```python
from build123d import *


with BuildPart() as f1:
    # F0 (on Front) → F1 (revolve)
    with BuildSketch(Plane.XZ):
        Polygon((0, 3.0734), (0, 0), (25.4, 0), (46.035527, 41.271053), (46.613301, 42.426601), (47.191074, 43.582149), (47.685844, 44.571688), (50.8, 50.8), (47.363834, 50.8), (23.500534, 3.0734), align=None)
        Polygon((47.191074, 43.582149), (46.613301, 42.426601), (47.191074, 42.426601), align=None)
        Polygon((47.685844, 44.571688), (47.191074, 43.582149), (47.685844, 43.582149), align=None)
        Polygon((46.613301, 42.426601), (46.035527, 41.271053), (46.613301, 41.271053), align=None)
    revolve(axis=Axis((0, 0, 25.4), (0, 0, 1)))


solid = f1.part
```
Model file for the job. Use its own axes, mm. A direction names the side the tool comes from. Coordinates: 2 decimals unless noted, no trailing zeros. Write each loop counter-clockwise with the first axis right and the second up, starting at its lowest first coordinate (ties: lowest second). Pieces come first, ordered by that corner, then holes. Notation, with made-up numbers: (-14.75, -26.75) - (3.25, -26.75) arc R16 ccw to (3.25, -10.75) - close; hole circle Ø2 at (-36.75, -29.75). An arc over 180 degrees is marked (long way). One line per item, written item: value. Start each with the question number.
1. Tool access for faces 1 (the flat face through (0, 0, 3.073)), 2 (the flat face through (0, 0, 0)), 3 (the flat face through (45.7, 10.7, 42.427)): list every direction of +Z, -Z, +X, -X, +Y, -Y with a clear straight run to the whole face (end or side of a thin tool).
2. Slice it at A-A (y = 0). Write the cut outline in (x, z), plus the area to 3 significant figures.
3. Slice it at C-C (z = 28). Write the cut outline in (x, y).
4. Mould opens along X. For faces 4 (the cylindrical face through (25.059, 39.305, 41.857)), 5 (the conical face through (-5.92, -26.66, 10.69)), 6 (the flat face through (-42, 23, 50.8)) say: released by +X, released by -X, zero draft, split by the parting line, or undercut.
5. Flat gauge pins, fed straight in: pin 1 (4 mm diameter, centred on x = -34, y = 20.5, fed in from +Z); pin 2 (5 mm diameter, centred on x = 7, y = -18.5, fed in from -Z); pin 3 (8 mm diameter, centred on y = -29, z = 16, fed in from +X); pin 4 (3 mm diameter, centred on y = 6.5, z = 7.5, fed in from +X). Where does each tip first touch, or does it go through?
6. Slice it at D-D (z = 46.5). Write the cut outline in (x, y), plus the area to 3 significant figures.
7. Probe line 1 (Y direction, x = 25, z = 47); line 2 (X direction, y = 10, z = 28.5); line 3 (X direction, y = 3, z = 38.5). List the from-to ranges inside material, lowest first. Write a range as from..to.
Answers below:
1. face 1: +Z
1. face 2: -Z, +X, -X, +Y, -Y
1. face 3: -Z
2. outline: (-50.8, 50.8) - (-47.69, 44.57) - (-47.69, 43.58) - (-47.19, 43.58) - (-47.19, 42.43) - (-46.61, 42.43) - (-46.61, 41.27) - (-46.04, 41.27) - (-25.4, 0) - (25.4, 0) - (46.04, 41.27) - (46.61, 41.27) - (46.61, 42.43) - (47.19, 42.43) - (47.19, 43.58) - (47.69, 43.58) - (47.69, 44.57) - (50.8, 50.8) - (47.36, 50.8) - (23.5, 3.07) - (-23.5, 3.07) - (-47.36, 50.8) - close
2. area: 491 mm^2
3. outline: circle Ø78.8 at (0, 0); hole circle Ø71.93 at (0, 0)
4. face 4: split by the parting line
4. face 5: undercut
4. face 6: zero draft
5. pin 1: stops at z = 39.48
5. pin 2: stops at z = 0
5. pin 3: stops at x = 23.06
5. pin 4: stops at x = 29.25
6. outline: circle Ø97.3 at (0, 0); hole circle Ø90.43 at (0, 0)
6. area: 1,010 mm^2
7. line 1: y = -42.03..-37.97, 37.97..42.03
7. line 2: x = -38.37..-34.81, 34.81..38.37
7. line 3: x = -44.55..-41.1, 41.1..44.55
